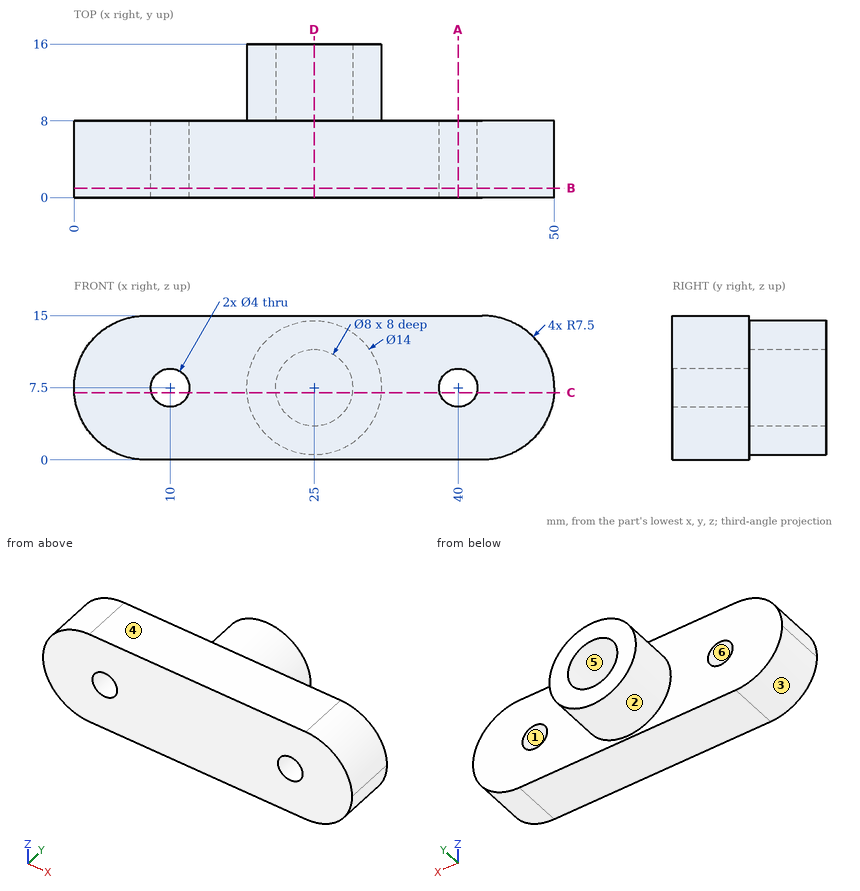
The figure shows three views and two pictorial views of one solid part (mm, origin at its lowest corner). Answer the questions. A direction names the side the tool comes from. Coordinates: 2 decimals unless noted, no trailing zeros. Loops run counter-clockwise (first coordinate to the right, second up) from the corner with the lowest first, then second, coordinate; pieces in that order, holes last. Notation, with made-up numbers: M 13.5,-31 L 42.5,-31 A24 cw 42.5,-2 Z; hole C -25.5,-5.5 d9. An arc over 180 degrees is marked long. Answer as CSV lines item,"result". Start each with the question number.
(1) For the marked faces 5 and 6, determine the directions among +Z, -Z, +X, -X, +Y, -Y from which every point of the face is accessible in a straight line to the end or side of a thin tool.
(2) The part is cut by section A-A (x = 40). Give the vertices of the cut face in (y, z), and give its area (3 significant figures).
(3) Given pin 1 (3 mm diameter, centred on x = 40, z = 7.5, fed in from -Y); pin 2 (6.5 mm diameter, centred on x = 25.5, z = 9, fed in from +Y); pin 3 (4 mm diameter, centred on x = 32, y = 13, fed in from -Z); pin 4 (3 mm diameter, centred on x = 26, y = 12.5, fed in from -Z), each flat-ended and moving along its own axis, determine where each tip first touches the part or whether it passes through.
(4) The part is cut by section B-B (y = 1). State how many separate pieces and enclosed holes the cut face has, and give its area (3 significant figures).
(5) The mould has two halves that part along Z. Classify the marked faces 1, 2, 3 and 4: pulls with the +Z half, pulls with the -Z half, needs draft (parallel to the pull), parting line crosses it, or undercut.
(6) The part is cut by section D-D (x = 25). Give the vertices of the cut face in (y, z), and give its area (3 significant figures).
(7) Find the intervals of material crossed by L1, parallel to X at y = 2, z = 7.5; L2, parallel to X at y = 10.25, z = 7.25; L3, parallel to Y at x = 48, z = 12.5, in increasing order. Write a range as [from, to].
(8) The part is cut by section C-C (z = 7). Give the vertices of the cut face in (x, y), and give its area (3 significant figures).
Determined:
1,face 5,"+Y"
1,face 6,"+Y, -Y"
2,outline,"M 0,0 L 8,0 L 8,5.5 L 0,5.5 Z; M 0,9.5 L 8,9.5 L 8,15 L 0,15 Z"
2,area,"88.0 mm2"
3,pin 1,"through"
3,pin 2,"y = 16"
3,pin 3,"z = 2.6"
3,pin 4,"z = 0.5"
4,separate pieces,"1"
4,enclosed holes,"2"
4,area,"677 mm2"
5,face 1,"undercut"
5,face 2,"parting line crosses it"
5,face 3,"pulls with the -Z half"
5,face 4,"pulls with the +Z half"
6,outline,"M 0,0 L 8,0 L 8,0.5 L 16,0.5 L 16,3.5 L 8,3.5 L 8,11.5 L 16,11.5 L 16,14.5 L 8,14.5 L 8,15 L 0,15 Z"
6,area,"168 mm2"
7,L1,"[0, 8], [12, 38], [42, 50]"
7,L2,"[18, 21.01], [28.99, 32]"
7,L3,"[0, 8]"
8,outline,"M 0.02,0 L 8.06,0 L 8.06,8 L 0.02,8 Z; M 11.94,0 L 38.06,0 L 38.06,8 L 31.98,8 L 31.98,16 L 28.97,16 L 28.97,8 L 21.03,8 L 21.03,16 L 18.02,16 L 18.02,8 L 11.94,8 Z; M 41.94,0 L 49.98,0 L 49.98,8 L 41.94,8 Z"
8,area,"386 mm2"
